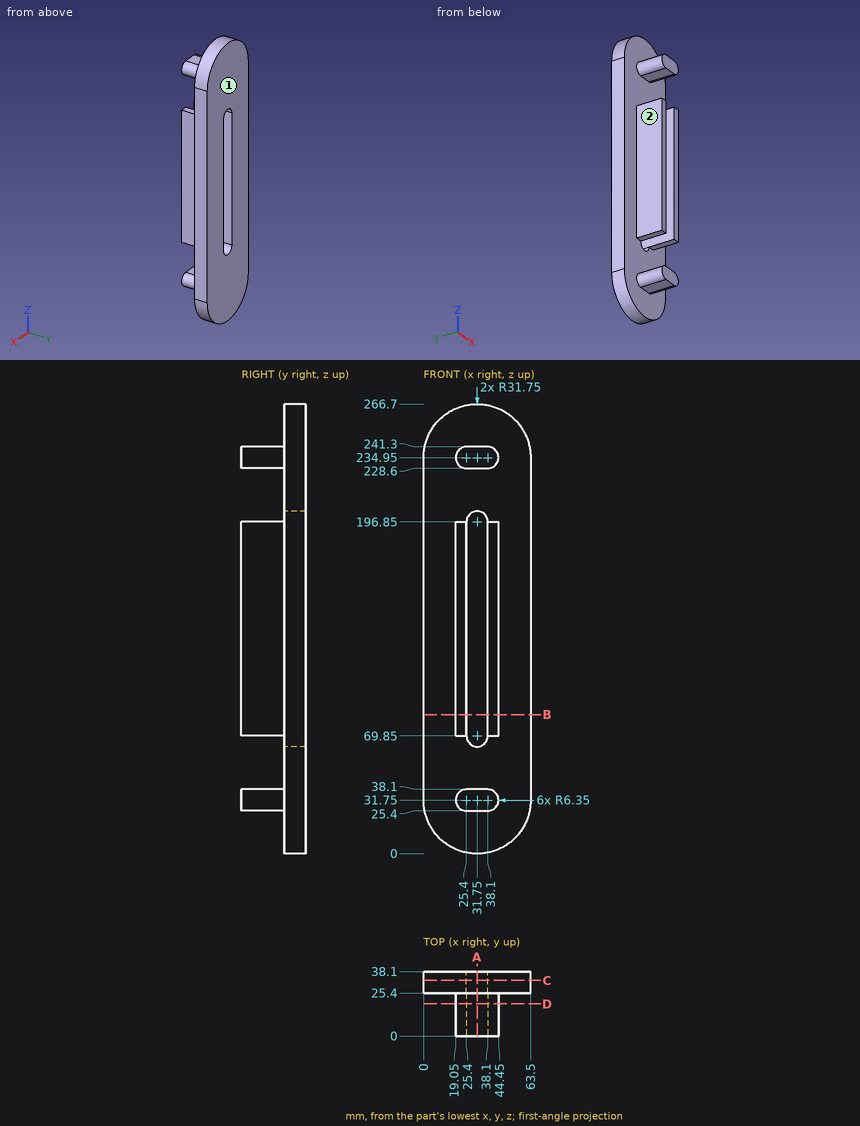
The figure shows three views and two pictorial views of one solid part (mm, origin at its lowest corner). Answer the questions. A direction names the side the tool comes from. Give positions to 0.01 mm unless a question says otherwise; leave off trailing zeros. Write each loop counter-clockwise with the first axis right and the second up, starting at its lowest first coordinate (ties: lowest second). Pieces come first, ordered by that corner, then holes. Notation, with made-up numbers: (15, -20.75) - (25, -20.75) arc R16 ccw to (25, -3.75) - close; hole circle Ø7 at (25, -5.5). An arc over 180 degrees is marked (long way). Use one line per item in the form item = value. Start each with the question number.
1) Flat-ended cylindrical pins translate along their axes: pin 1 Ø14 at (x, y) = (32, 8) entering from +Z; pin 2 Ø12 at (x, y) = (9.5, 34) entering from -Z; pin 3 Ø3 at (y, z) = (22, 105) entering from +X. Find the tip coordinate at first contact, or state that the pin passes through.
2) Consider line 1 along X through (y, z) = (7.5, 152); line 2 along Z through (x, y) = (39.5, 13); line 3 along Z through (x, y) = (35, 12). Determine where each line is inside the solid, lowest interval first. Write a range as from..to.
3) A tool of negligible diameter and unlimited length cuts with its end or side. For the marked faces 1 and 2, from which of +Z, -Z, +X, -X, +Y, -Y can it reach the whole face along a straight path? Write none if from no direction.
4) Find section C-C on y = 33. Determine the outline of the cut face in (x, z).
5) Find section A-A on x = 31.75. Determine the outline of the cut face in (y, z).
6) Find section B-B on z = 82.5. Determine the outline of the cut face in (x, y), plus the area to 3 significant figures.
7) Find section D-D on y = 19. Determine the outline of the cut face in (x, z).
Geometry results:
q1.pin_1 = 241.3
q1.pin_2 = 4.47
q1.pin_3 = 44.45
q2.line_1 = 19.05..25.4, 38.1..44.45
q2.line_2 = 25.56..37.94, 69.85..196.85, 228.76..241.14
q2.line_3 = 25.4..38.1, 228.6..241.3
q3.face_1 = +Z, -Z, +X, -X, +Y
q3.face_2 = +Z, -Z, -X, -Y
q4.outline = (0, 31.75) arc R31.75 ccw to (63.5, 31.75) - (63.5, 234.95) arc R31.75 ccw to (0, 234.95) - close; hole (25.4, 69.85) arc R6.35 ccw to (38.1, 69.85) - (38.1, 196.85) arc R6.35 ccw to (25.4, 196.85) - close
q5.outline = (0, 25.4) - (25.4, 25.4) - (25.4, 0) - (38.1, 0) - (38.1, 63.5) - (25.4, 63.5) - (25.4, 38.1) - (0, 38.1) - close; (0, 228.6) - (25.4, 228.6) - (25.4, 203.2) - (38.1, 203.2) - (38.1, 266.7) - (25.4, 266.7) - (25.4, 241.3) - (0, 241.3) - close
q6.outline = (0, 25.4) - (19.05, 25.4) - (19.05, 0) - (25.4, 0) - (25.4, 38.1) - (0, 38.1) - close; (38.1, 0) - (44.45, 0) - (44.45, 25.4) - (63.5, 25.4) - (63.5, 38.1) - (38.1, 38.1) - close
q6.area = 968 mm2
q7.outline = (19.05, 69.85) - (25.4, 69.85) - (25.4, 196.85) - (19.05, 196.85) - close; (25.4, 25.4) - (38.1, 25.4) arc R6.35 ccw to (38.1, 38.1) - (25.4, 38.1) arc R6.35 ccw to start; (25.4, 228.6) - (38.1, 228.6) arc R6.35 ccw to (38.1, 241.3) - (25.4, 241.3) arc R6.35 ccw to start; (38.1, 69.85) - (44.45, 69.85) - (44.45, 196.85) - (38.1, 196.85) - close
